Could you check a few things on this drawing? It's one solid part, dimensions in mm from its lowest x, y, z. Give positions to 0.01 mm unless a question says otherwise; leave off trailing zeros. Order: outer loops, then holes, each group sorted by start corner. A loop starts at its lowest first (then second) coordinate and runs counter-clockwise, first axis right, second up. Notation, with made-up numbers: (-36, -11.75) -> (-6, -11.75) arc R17 cw to (-6, -1.75) -> close; hole circle Ø4 at (-16.75, 20). An arc over 180 degrees is marked (long way). Use one line per item in the form item = value. Start each with the question number.
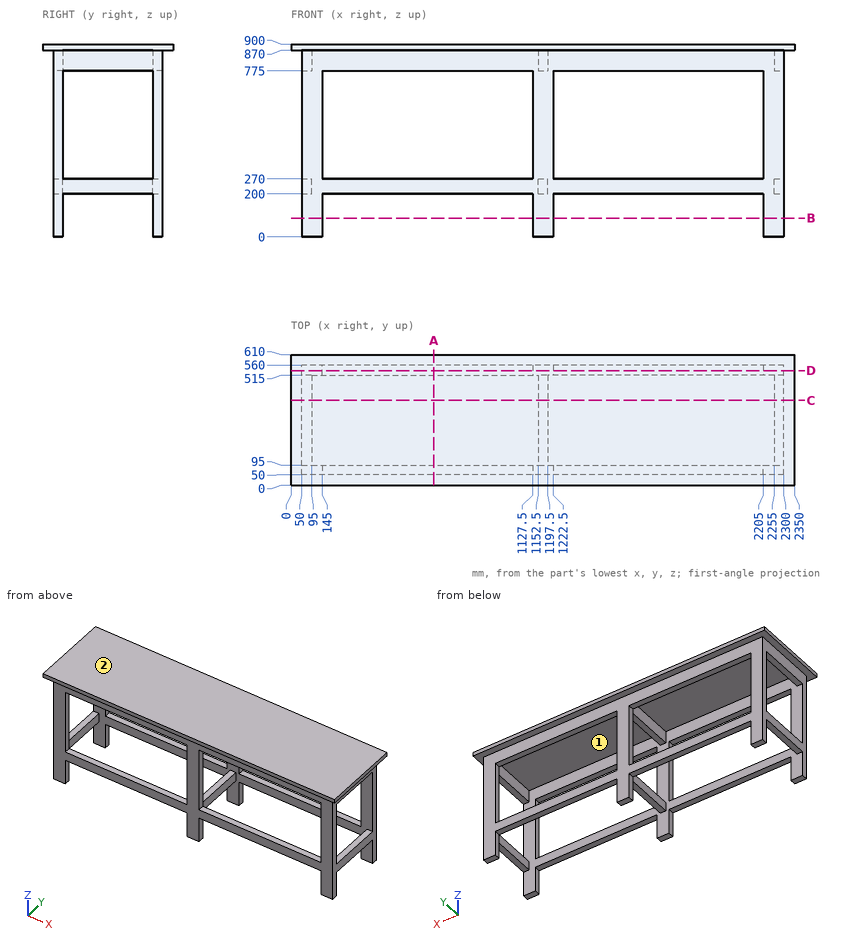
(1) Imagine slicing it at D-D (y = 536.5). Write out the boundary of the cut face in (x, z), plus the area to 3 significant figures.
(2) I'm going to push flat-ended pins straight in: pin 1 Ø21 at (y, z) = (247.5, 249) entering from +X; pin 2 Ø22.5 at (x, y) = (528.5, 534) entering from -Z; pin 3 Ø5 at (x, y) = (1784.5, 425.5) entering from -Z. Where does each tip first touch, or does it pass through?
(3) We'd pull the mould along X, two halves only. Please class the marked faces 1 and 2: pulls with the +X half, pulls with the -X half, needs draft (parallel to the pull), parting line crosses it, or undercut.
(4) Imagine slicing it at C-C (y = 397.5). Write out the boundary of the cut face in (x, z).
(5) Imagine slicing it at B-B (z = 87). Write out the boundary of the cut face in (x, y), plus the area to 4 significant figures.
(6) Imagine slicing it at A-A (x = 666.5). Write out the boundary of the cut face in (y, z).
(7) Please list where these lines run through material, in increasing order: probe 1 along X at (y, z) = (431, 824); probe 2 along X at (y, z) = (58.5, 42); probe 3 along Y at (x, z) = (1932.5, 218).
Calculated:
q1.outline = (0, 870) -> (50, 870) -> (50, 0) -> (145, 0) -> (145, 200) -> (1127.5, 200) -> (1127.5, 0) -> (1222.5, 0) -> (1222.5, 200) -> (2205, 200) -> (2205, 0) -> (2300, 0) -> (2300, 870) -> (2350, 870) -> (2350, 900) -> (0, 900) -> close; hole (145, 270) -> (1127.5, 270) -> (1127.5, 775) -> (145, 775) -> close; hole (1222.5, 270) -> (2205, 270) -> (2205, 775) -> (1222.5, 775) -> close
q1.area = 643,000 mm2
q2.pin_1 = 2300
q2.pin_2 = 200
q2.pin_3 = 870
q3.face_1 = undercut
q3.face_2 = needs draft
q4.outline = (0, 870) -> (50, 870) -> (50, 775) -> (95, 775) -> (95, 870) -> (1152.5, 870) -> (1152.5, 775) -> (1197.5, 775) -> (1197.5, 870) -> (2255, 870) -> (2255, 775) -> (2300, 775) -> (2300, 870) -> (2350, 870) -> (2350, 900) -> (0, 900) -> close; (50, 200) -> (95, 200) -> (95, 270) -> (50, 270) -> close; (1152.5, 200) -> (1197.5, 200) -> (1197.5, 270) -> (1152.5, 270) -> close; (2255, 200) -> (2300, 200) -> (2300, 270) -> (2255, 270) -> close
q5.outline = (50, 50) -> (145, 50) -> (145, 95) -> (50, 95) -> close; (50, 515) -> (145, 515) -> (145, 560) -> (50, 560) -> close; (1127.5, 50) -> (1222.5, 50) -> (1222.5, 95) -> (1127.5, 95) -> close; (1127.5, 515) -> (1222.5, 515) -> (1222.5, 560) -> (1127.5, 560) -> close; (2205, 50) -> (2300, 50) -> (2300, 95) -> (2205, 95) -> close; (2205, 515) -> (2300, 515) -> (2300, 560) -> (2205, 560) -> close
q5.area = 25,650 mm2
q6.outline = (0, 870) -> (50, 870) -> (50, 775) -> (95, 775) -> (95, 870) -> (515, 870) -> (515, 775) -> (560, 775) -> (560, 870) -> (610, 870) -> (610, 900) -> (0, 900) -> close; (50, 200) -> (95, 200) -> (95, 270) -> (50, 270) -> close; (515, 200) -> (560, 200) -> (560, 270) -> (515, 270) -> close
q7.probe_1 = 50 to 95, 1152.5 to 1197.5, 2255 to 2300
q7.probe_2 = 50 to 145, 1127.5 to 1222.5, 2205 to 2300
q7.probe_3 = 50 to 95, 515 to 560
